from build123d import *

# Parameters (mm, degrees)
SKETCH1_W           = 8
SKETCH1_H           = 8
BOSS_EXTRUDE1_DEPTH = 8
SKETCH2_W           = 3.9
SKETCH2_H           = 3.8
BOSS_EXTRUDE2_DEPTH = 2.4
SKETCH3_W           = 2
SKETCH3_H           = 3
BOSS_EXTRUDE3_DEPTH = 3
SKETCH4_W           = 1
SKETCH4_H           = 1
BOSS_EXTRUDE4_DEPTH = 3.6
SKETCH5_W           = 0.5
SKETCH5_H           = 1
CUT_EXTRUDE1_DEPTH  = 15.851262573


with BuildPart() as part:
    # Sketch1 → Boss-Extrude1 (new body)
    with BuildSketch(Plane(origin=(0, 0, 0), x_dir=(1, 0, 0), z_dir=(0, 1, 0))):
        Rectangle(SKETCH1_W, SKETCH1_H)
    extrude(amount=BOSS_EXTRUDE1_DEPTH)

    # Sketch2 → Boss-Extrude2 (add)
    with BuildSketch(Plane(origin=(0, 8, 0), x_dir=(1, 0, 0), z_dir=(0, 1, 0))):
        Rectangle(SKETCH2_W, SKETCH2_H)
    extrude(amount=BOSS_EXTRUDE2_DEPTH)

    # Sketch3 → Boss-Extrude3 (add)
    with BuildSketch(Plane(origin=(0, 10.4, 0), x_dir=(1, 0, 0), z_dir=(0, 1, 0))):
        Rectangle(SKETCH3_W, SKETCH3_H)
    extrude(amount=BOSS_EXTRUDE3_DEPTH)

    # Sketch4 → Boss-Extrude4 (add)
    with BuildSketch(Plane.XZ):
        with Locations((0, 2.5)):
            Rectangle(SKETCH4_W, SKETCH4_H)
        with Locations((-2, 2.5)):
            Rectangle(SKETCH4_W, SKETCH4_H)
        with Locations((2, 2.5)):
            Rectangle(SKETCH4_W, SKETCH4_H)
        with Locations((0, -2.5)):
            Rectangle(SKETCH4_W, SKETCH4_H)
        with Locations((2, -2.5)):
            Rectangle(SKETCH4_W, SKETCH4_H)
        with Locations((-2, -2.5)):
            Rectangle(SKETCH4_W, SKETCH4_H)
    extrude(amount=BOSS_EXTRUDE4_DEPTH)

    # Sketch5 → Cut-Extrude1 (cut, through all)
    with BuildSketch(Plane(origin=(1, 0, 0), x_dir=(0, 0, -1), z_dir=(1, 0, 0))):
        with Locations((-1.25, 11.9)):
            Rectangle(SKETCH5_W, SKETCH5_H)
        with Locations((1.25, 11.9)):
            Rectangle(SKETCH5_W, SKETCH5_H)
    extrude(amount=-CUT_EXTRUDE1_DEPTH, mode=Mode.SUBTRACT)


solid = part.part
The listing builds one solid part. Answer for the finished solid, in the listing's coordinates (mm). A direction names the side the tool comes from. Coordinates: 2 decimals unless noted, no trailing zeros. Write each loop counter-clockwise with the first axis right and the second up, starting at its lowest first coordinate (ties: lowest second). Pieces come first, ordered by that corner, then holes. Notation, with made-up numbers: M 81.25,24 L 96.25,24 A26 cw 96.25,44 Z; hole C 60,82 d7. An arc over 180 degrees is marked long. Put each result on its own line as item: value. Start each with the question number.
1. A cutting plane is placed at D-D on y = 9.75. Write down the section's boundary in (x, z), then the cut area to 3 significant figures.
2. For a pull along X with two mould halves and no side action, classify faces 4 (the flat face through (-1.3, 10.4, 0)), 5 (the flat face through (2.5, -1.8, 2.5)), 6 (the flat face through (-0.5, -1.8, -2.5)) as pulls with the +X half, pulls with the -X half, needs draft (parallel to the pull), parting line crosses it, or undercut.
3. A cutting plane is placed at C-C on z = 1.25. Write down the section's boundary in (x, y), then the cut area to 3 significant figures.
4. A cutting plane is placed at B-B on x = 0. Write down the section's boundary in (y, z), then the cut area to 3 significant figures.
5. A cutting plane is placed at A-A on y = -1. Write down the section's boundary in (x, z), then the cut area to 3 significant figures.
6. Flat-ended cylindrical pins translate along their axes: P1, Ø1.1, axis at y = -2, z = -2.5, coming from the +X side; P2, Ø0.6, axis at x = 0.5, z = -1.5, coming from the -Y side; P3, Ø0.8, axis at x = -2, y = -2.5, coming from the +Z side. Find the tip coordinate at first contact, or state that the pin passes through.
7. Consider line 1 (Z direction, x = 1, y = 10.25); line 2 (Y direction, x = 0.75, z = 3.5); line 3 (Z direction, x = 0.5, y = 12). Determine where each line is inside the solid, lowest interval first. Write a range as from..to.
8. Which of the six approach directions +Z, -Z, +X, -X, +Y, -Y give full straight-line access (tool end or side, diameter ignored) to faces 1 (the flat face through (2, -2, -3)), 2 (the flat face through (1.5, -1.8, 2.5)), 3 (the flat face through (0, -2, -2))?
Resolved:
1. outline: M -1.95,-1.9 L 1.95,-1.9 L 1.95,1.9 L -1.95,1.9 Z
1. area: 14.8 mm2
2. face 4: needs draft
2. face 5: pulls with the +X half
2. face 6: undercut
3. outline: M -4,0 L 4,0 L 4,8 L 1.95,8 L 1.95,10.4 L 1,10.4 L 1,11.4 L -1,11.4 L -1,10.4 L -1.95,10.4 L -1.95,8 L -4,8 Z; M -1,12.4 L 1,12.4 L 1,13.4 L -1,13.4 Z
3. area: 77.4 mm2
4. outline: M -3.6,-3 L 0,-3 L 0,-4 L 8,-4 L 8,-1.9 L 10.4,-1.9 L 10.4,-1.5 L 11.4,-1.5 L 11.4,-1 L 12.4,-1 L 12.4,-1.5 L 13.4,-1.5 L 13.4,1.5 L 12.4,1.5 L 12.4,1 L 11.4,1 L 11.4,1.5 L 10.4,1.5 L 10.4,1.9 L 8,1.9 L 8,4 L 0,4 L 0,3 L -3.6,3 L -3.6,2 L 0,2 L 0,-2 L -3.6,-2 Z
4. area: 88.3 mm2
5. outline: M -2.5,-3 L -1.5,-3 L -1.5,-2 L -2.5,-2 Z; M -2.5,2 L -1.5,2 L -1.5,3 L -2.5,3 Z; M -0.5,-3 L 0.5,-3 L 0.5,-2 L -0.5,-2 Z; M -0.5,2 L 0.5,2 L 0.5,3 L -0.5,3 Z; M 1.5,-3 L 2.5,-3 L 2.5,-2 L 1.5,-2 Z; M 1.5,2 L 2.5,2 L 2.5,3 L 1.5,3 Z
5. area: 6.00 mm2
6. P1: stops at x = 2.5
6. P2: stops at y = 0
6. P3: stops at z = 3
7. line 1: z = -1.9..1.9
7. line 2: y = 0..8
7. line 3: z = -1..1
8. face 1: -Z, +X, -X, -Y
8. face 2: +Z, -Z, -Y
8. face 3: +X, -X, -Y
